Part model, mm, in its own coordinate system. Face numbers are marked on the shaded views. A direction names the side the tool comes from. Round coordinates to 2 decimals unless told otherwise and drop trailing zeros. Loops run counter-clockwise (first coordinate to the right, second up) from the corner with the lowest first, then second, coordinate; pieces in that order, holes last. Notation, with made-up numbers: (-6, 0) - (1, 0) arc R29 ccw to (1, 21) - close; hole circle Ø10 at (14, -36). An arc over 180 degrees is marked (long way). Put each result on its own line as item: value.
from build123d import *

# Parameters (mm, degrees)
CYLINDER085_R     = 2.75
CYLINDER085_DEPTH = 7
CYLINDER084_R     = 4
CYLINDER084_DEPTH = 9
CYLINDER073_R     = 1.38
CYLINDER073_DEPTH = 10
CYLINDER074_R     = 2.25
CYLINDER074_DEPTH = 10
BOX041_W          = 25
BOX041_H          = 10
BOX041_DEPTH      = 4
FILLET008_R       = 3


with BuildPart() as cilindro004:
    # Cylinder085 → Cylinder085 (new body)
    with BuildSketch(Plane(origin=(17, 17, 12), x_dir=(1, 0, 0), z_dir=(0, 0, 1))):
        Circle(CYLINDER085_R)
    extrude(amount=CYLINDER085_DEPTH)


with BuildPart() as obj1:
    # Cylinder084 → Cylinder084 (new body)
    with BuildSketch(Plane(origin=(17, 17, 10), x_dir=(1, 0, 0), z_dir=(0, 0, 1))):
        Circle(CYLINDER084_R)
    extrude(amount=CYLINDER084_DEPTH)

    # Cut055: cut Cilindro004
    add(cilindro004.part, mode=Mode.SUBTRACT)


with BuildPart() as obj1_1:
    # Cut055 placement: moved
    add(obj1.part.moved(Location((21, 102, 52))))


with BuildPart() as cylinder073:
    # Cylinder073 → Cylinder073 (new body)
    with BuildSketch(Plane(origin=(25, 52, 59), x_dir=(1, 0, 0), z_dir=(0, 0, 1))):
        Circle(CYLINDER073_R)
    extrude(amount=CYLINDER073_DEPTH)


with BuildPart() as cylinder074:
    # Cylinder074 → Cylinder074 (new body)
    with BuildSketch(Plane(origin=(40, 52, 59), x_dir=(1, 0, 0), z_dir=(0, 0, 1))):
        Circle(CYLINDER074_R)
    extrude(amount=CYLINDER074_DEPTH)


with BuildPart() as palanca_3_final:
    # Box041 → Box041 (new body)
    with BuildSketch(Plane(origin=(45, 57, 62), x_dir=(-1, 0, 0), z_dir=(0, 0, 1))):
        with Locations((12.5, 5)):
            Rectangle(BOX041_W, BOX041_H)
    extrude(amount=BOX041_DEPTH)

    # Cut044: cut Cylinder074
    add(cylinder074.part, mode=Mode.SUBTRACT)

    # Cut045: cut Cylinder073
    add(cylinder073.part, mode=Mode.SUBTRACT)

    # Fillet008
    fillet008_edges = [palanca_3_final.edges().sort_by_distance(p)[0] for p in [
        (20, 57, 64),
        (20, 47, 64),
    ]]
    fillet(fillet008_edges, radius=FILLET008_R)


with BuildPart() as palanca_3_final_1:
    # Fillet008 placement: moved
    add(palanca_3_final.part.moved(Location((-2, 67, 0))))

    # Fusion011: union obj1
    add(obj1_1.part)


solid = palanca_3_final_1.part
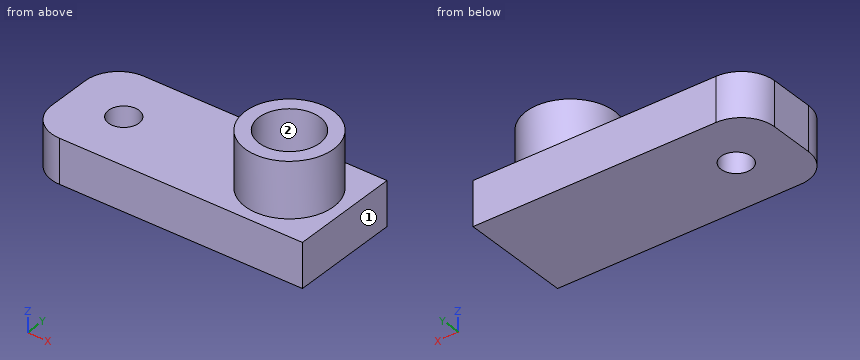
1. Band-saw the part on C-C (y = 119). List the corners of the cut face in (x, z).
A:
outline: (18, 62) - (21.62, 62) - (21.62, 66) - (18, 66) - close; (24.38, 62) - (43, 62) - (43, 66) - (42, 66) - (42, 71) - (40.75, 71) - (40.75, 66) - (40.25, 66) - (40.25, 64) - (35.75, 64) - (35.75, 66) - (35.25, 66) - (35.25, 71) - (34, 71) - (34, 66) - (24.38, 66) - close
2. Pin check, flat tips, straight feed: P1, Ø2.5, axis at x = 23, y = 119, coming from the -Z side; P2, Ø5, axis at x = 38, y = 119, coming from the +Z side. Stop position of each tip, or through.
A:
P1: passes through
P2: stops at z = 66
3. Band-saw the part on D-D (z = 65.75). List the corners of the cut face in (x, y), plus the area to 3 significant figures.
A:
outline: (18, 117) arc R3 ccw to (21, 114) - (43, 114) - (43, 124) - (21, 124) arc R3 ccw to (18, 121) - close; hole circle Ø2.76 at (23, 119); hole circle Ø4.5 at (38, 119)
area: 224 mm²
4. Probe line 1 along X through (y, z) = (119, 64.05); line 2 along Y through (x, z) = (38, 67.25); line 3 along Y through (x, z) = (38, 65.45). List the from-to ranges inside material, lowest first. Write a range as [from, to].
A:
line 1: x = [18, 21.62], [24.38, 35.75], [40.25, 43]
line 2: y = [115, 116.25], [121.75, 123]
line 3: y = [114, 116.75], [121.25, 124]
5. Band-saw the part on B-B (z = 63). List the corners of the cut face in (x, y), plus the area to 3 significant figures.
A:
outline: (18, 117) arc R3 ccw to (21, 114) - (43, 114) - (43, 124) - (21, 124) arc R3 ccw to (18, 121) - close; hole circle Ø2.76 at (23, 119)
area: 240 mm²
6. Band-saw the part on A-A (x = 23). List the corners of the cut face in (y, z), plus the area to 3 significant figures.
A:
outline: (114, 62) - (117.62, 62) - (117.62, 66) - (114, 66) - close; (120.38, 62) - (124, 62) - (124, 66) - (120.38, 66) - close
area: 29.0 mm²
7. Tool access for the marked faces 1 and 2: list every direction of +Z, -Z, +X, -X, +Y, -Y with a clear straight run to the whole face (end or side of a thin tool).
A:
face 1: +Z, -Z, +X, +Y, -Y
face 2: +Z
